Here's how the part is built. I have some questions about the finished solid (model axes, mm). Coordinates: 2 decimals unless noted, no trailing zeros. Loops run counter-clockwise (first coordinate to the right, second up) from the corner with the lowest first, then second, coordinate; pieces in that order, holes last. Notation, with made-up numbers: (-29, 56.25) -> (-9, 56.25) arc R14 cw to (-9, 70.25) -> close; hole circle Ø2 at (28, 59.25). An arc over 180 degrees is marked (long way). Use CSV: the item, a comma, the result in double quotes. Start each with the question number.
from build123d import *

# Parameters (mm, degrees)
F0_R     = 1
F0_R_2   = 5
F0_R_3   = 2
F1_DEPTH = 1.5


with BuildPart() as f1:
    # F0 (on Top) → F1 (new body)
    with BuildSketch(Plane.XY):
        with BuildLine():
            Line((9.062422, 2.85), (3.338787, 21.05))
            ThreePointArc((3.338787, 21.05), (0, 23.5), (-3.338787, 21.05))
            Line((-3.338787, 21.05), (-9.062422, 2.85))
            ThreePointArc((-9.062422, 2.85), (0, -9.5), (9.062422, 2.85))
        make_face()
        with Locations((-4.949747, -4.949747)):
            Circle(F0_R, mode=Mode.SUBTRACT)
        with Locations((-7, 0)):
            Circle(F0_R, mode=Mode.SUBTRACT)
        with Locations((-4.949747, 4.949747)):
            Circle(F0_R, mode=Mode.SUBTRACT)
        with Locations((0, -7)):
            Circle(F0_R, mode=Mode.SUBTRACT)
        with Locations((4.949747, -4.949747)):
            Circle(F0_R, mode=Mode.SUBTRACT)
        Circle(F0_R_2, mode=Mode.SUBTRACT)
        with Locations((7, 0)):
            Circle(F0_R, mode=Mode.SUBTRACT)
        with Locations((4.949747, 4.949747)):
            Circle(F0_R, mode=Mode.SUBTRACT)
        with Locations((0, 7)):
            Circle(F0_R, mode=Mode.SUBTRACT)
        with Locations((0, 20)):
            Circle(F0_R_3, mode=Mode.SUBTRACT)
    extrude(amount=F1_DEPTH)


solid = f1.part
1) Please list where these lines run through material, in increasing order: L1, parallel to Y at x = 0, z = 0.85; L2, parallel to X at y = 21.5, z = 1.45; L3, parallel to Y at x = -2.25, z = 1.4. Write a range as [from, to].
2) I want a section at B-B, the plane y = -3. Please give me the cut outline in (x, z).
3) I want a section at C-C, the plane x = 7. Please give me the cut outline in (y, z), plus the area to 3 significant figures.
4) For P1, Ø1.8, axis at x = 4.95, y = -4.95, coming from the -Z side, with a flat end and sliding along its axis, tell me the tip position at first contact or that it passes through.
5) I want a section at A-A, the plane x = 0. Please give me the cut outline in (y, z), plus the area to 3 significant figures.
6) I want a section at D-D, the plane z = 0.65. State how many separate pieces and enclosed holes the cut face has, plus the area to 3 significant figures.
Return value:
1,L1,"y = [-9.5, -8], [-6, -5], [5, 6], [8, 18], [22, 23.5]"
1,L2,"x = [-3.16, -1.32], [1.32, 3.16]"
1,L3,"y = [-9.23, -4.47], [4.47, 22.68]"
2,outline,"(-9.01, 0) -> (-4, 0) -> (-4, 1.5) -> (-9.01, 1.5) -> close; (4, 0) -> (9.01, 0) -> (9.01, 1.5) -> (4, 1.5) -> close"
3,outline,"(-6.42, 0) -> (-1, 0) -> (-1, 1.5) -> (-6.42, 1.5) -> close; (1, 0) -> (9.41, 0) -> (9.41, 1.5) -> (1, 1.5) -> close"
3,area,"20.7 mm²"
4,P1,"passes through"
5,outline,"(-9.5, 0) -> (-8, 0) -> (-8, 1.5) -> (-9.5, 1.5) -> close; (-6, 0) -> (-5, 0) -> (-5, 1.5) -> (-6, 1.5) -> close; (5, 0) -> (6, 0) -> (6, 1.5) -> (5, 1.5) -> close; (8, 0) -> (18, 0) -> (18, 1.5) -> (8, 1.5) -> close; (22, 0) -> (23.5, 0) -> (23.5, 1.5) -> (22, 1.5) -> close"
5,area,"22.5 mm²"
6,separate pieces,"1"
6,enclosed holes,"10"
6,area,"317 mm²"
